Work out the finished part from the listing and answer in its coordinate system (mm). A direction names the side the tool comes from. Round coordinates to 2 decimals unless told otherwise and drop trailing zeros. Order: outer loops, then holes, each group sorted by start corner. A loop starts at its lowest first (then second) coordinate and runs counter-clockwise, first axis right, second up. Notation, with made-up numbers: (24.5, -4) - (74.5, -4) arc R24 cw to (74.5, 25) - close; hole circle Ø5 at (85.5, 71.5). An arc over 180 degrees is marked (long way). Answer in a Markdown table with one row per item.
from build123d import *

# Parameters (mm, degrees)
F0_R     = 37.5
F1_DEPTH = 25
F4_R     = 12.5
F5_DEPTH = 25
F7_DEPTH = 25


with BuildPart() as f1:
    # F0 (on Front) → F1 (new body)
    with BuildSketch(Plane.XZ):
        Circle(F0_R)
    extrude(amount=F1_DEPTH)

    # F4 (on face) → F5 (cut)
    with BuildSketch(Plane.XZ.offset(25)):
        with Locations((-2.5, 7.5)):
            Circle(F4_R)
    extrude(amount=-F5_DEPTH, mode=Mode.SUBTRACT)

    # F6 (on face) → F7 (join)
    with BuildSketch(Plane.XZ.offset(25)):
        Polygon((1.973449, -23.717072), (12.871587, -23.717072), (16.239297, -13.352327), (7.422518, -6.946562), (-1.394261, -13.352327), align=None)
    extrude(amount=F7_DEPTH)


solid = f1.part
1) Find section C-C, the plane y = -7.5. Give the vertices of the cut face in (x, z).
Filled in:
| item | result |
|---|---|
| outline | circle Ø75 at (0, 0); hole circle Ø25 at (-2.5, 7.5) |
2) Find section D-D, the plane z = -15.5. Give the vertices of the cut face in (x, y), then the cut area to 3 significant figures.
Filled in:
| item | result |
|---|---|
| outline | (-34.15, -25) - (-0.7, -25) - (-0.7, -50) - (15.54, -50) - (15.54, -25) - (34.15, -25) - (34.15, 0) - (-34.15, 0) - close |
| area | 2,110 mm^2 |
3) Each of these flat-tipped pins is pushed along its axis until it touches: pin 1 (12 mm diameter, centred on x = 5.5, y = -41.5, fed in from -Z); pin 2 (8 mm diameter, centred on x = 4, y = -20.5, fed in from -Z); pin 3 (1 mm diameter, centred on y = -13.5, z = 22, fed in from +X). Where does it stop, or does it pass through?
Filled in:
| item | result |
|---|---|
| pin 1 | stops at z = -23.72 |
| pin 2 | stops at z = -37.5 |
| pin 3 | stops at x = 30.72 |
4) Find section A-A, the plane z = 0. Give the vertices of the cut face in (x, y), then the cut area to 4 significant figures.
Filled in:
| item | result |
|---|---|
| outline | (-37.5, -25) - (-12.5, -25) - (-12.5, 0) - (-37.5, 0) - close; (7.5, -25) - (37.5, -25) - (37.5, 0) - (7.5, 0) - close |
| area | 1,375 mm^2 |
5) Which of the six approach directions +Z, -Z, +X, -X, +Y, -Y give full straight-line access (tool end or side, diameter ignored) to faces 1 (the face through (3.08, -37.33, -10.1)), 2 (the face through (7, -37, -23.717)), 3 (the face through (0.266, -37.325, -18.462))?
Filled in:
| item | result |
|---|---|
| face 1 | +Z, -X, -Y |
| face 2 | -Z, +X, -X, -Y |
| face 3 | -Z, -X, -Y |
6) Find the intervals of material crossed by probe 1 along Y at (x, z) = (12.5, 4); probe 2 along X at (y, z) = (-16, 8); probe 3 along Z at (x, y) = (-10.5, -18), in increasing order. Write a range as from..to.
Filled in:
| item | result |
|---|---|
| probe 1 | y = -25..0 |
| probe 2 | x = -36.64..-14.99, 9.99..36.64 |
| probe 3 | z = -36..-2.1, 17.1..36 |
7) Find section B-B, the plane x = 0. Give the vertices of the cut face in (y, z), then the cut area to 3 significant figures.
Filled in:
| item | result |
|---|---|
| outline | (-50, -17.64) - (-25, -17.64) - (-25, -37.5) - (0, -37.5) - (0, -4.75) - (-25, -4.75) - (-25, -12.34) - (-50, -12.34) - close; (-25, 19.75) - (0, 19.75) - (0, 37.5) - (-25, 37.5) - close |
| area | 1,400 mm^2 |
